Source: CAD feature listing. Evaluate the final solid. Frame: model axes, mm. A direction names the side the tool comes from. Round coordinates to 2 decimals unless told otherwise and drop trailing zeros. Write each loop counter-clockwise with the first axis right and the second up, starting at its lowest first coordinate (ties: lowest second). Pieces come first, ordered by that corner, then holes. Notation, with made-up numbers: M 40.5,-21.5 L 71.5,-21.5 A33 cw 71.5,12.5 Z; hole C -4.5,43.25 d1. An arc over 180 degrees is marked long. Answer in a Markdown table with one row per item.
from build123d import *

# Parameters (mm, degrees)
BOSS_EXTRUDE1_DEPTH = 10
CUT_EXTRUDE1_REACH  = 3.5
SKETCH2_W           = 9
SKETCH2_H           = 5
CUT_EXTRUDE2_REACH  = 4


with BuildPart() as part:
    # Sketch1 → Boss-Extrude1 (new body)
    with BuildSketch(Plane(origin=(0, 0, 0), x_dir=(1, 0, 0), z_dir=(0, 1, 0))):
        Polygon((0, 0), (25.5, 0), (25.5, 11), (24, 11), (24, 2), (10, 2), (10, 14), (0, 14), align=None)
    extrude(amount=BOSS_EXTRUDE1_DEPTH)

    # Sketch2 → Cut-Extrude1 (cut, up to next)
    with BuildSketch(Plane.ZY.offset(-24), mode=Mode.PRIVATE) as cut_extrude1_sk1:
        with Locations((-6.5, 2.5)):
            Rectangle(SKETCH2_W, SKETCH2_H)
    cut_extrude1_tool1 = extrude(cut_extrude1_sk1.sketch, amount=-CUT_EXTRUDE1_REACH, mode=Mode.PRIVATE) & part.part
    add(cut_extrude1_tool1.solids().sort_by_distance((24, 2.5, -6.5))[0], mode=Mode.SUBTRACT)

    # Sketch3 → Cut-Extrude2 (cut, up to next)
    with BuildSketch(Plane(origin=(0, 0, -2), x_dir=(-1, 0, 0), z_dir=(0, 0, -1)), mode=Mode.PRIVATE) as cut_extrude2_sk1:
        with BuildLine():
            Line((-19.5, 5), (-14.5, 5))
            ThreePointArc((-14.5, 5), (-13, 3.5), (-14.5, 2))
            Line((-14.5, 2), (-19.5, 2))
            ThreePointArc((-19.5, 2), (-21, 3.5), (-19.5, 5))
        make_face()
    cut_extrude2_tool1 = extrude(cut_extrude2_sk1.sketch, amount=-CUT_EXTRUDE2_REACH, mode=Mode.PRIVATE) & part.part
    add(cut_extrude2_tool1.solids().sort_by_distance((17, 3.5, -2))[0], mode=Mode.SUBTRACT)


solid = part.part
Q1. Material intervals for probe 1 along X at (y, z) = (7.75, -4.25); probe 2 along Z at (x, y) = (22.75, 5); probe 3 along X at (y, z) = (4, -8.5), sorted ascending.
Solutions:
| item | result |
|---|---|
| probe 1 | x = 0 to 10, 24 to 25.5 |
| probe 2 | z = -2 to 0 |
| probe 3 | x = 0 to 10 |
Q2. Pull-direction query (Y, two-part tool) for faces 5 (the cylindrical face through (21, 3.5, -1)), 6 (the flat face through (7, 0, -7)), 7 (the flat face through (10, 5, -8)); classes: pulls with the +Y half, pulls with the -Y half, needs draft (parallel to the pull), parting line crosses it, or undercut.
Solutions:
| item | result |
|---|---|
| face 5 | undercut |
| face 6 | pulls with the -Y half |
| face 7 | needs draft |
Q3. Access query for faces 1 (the cylindrical face through (13, 3.5, -1)), 2 (the flat face through (25, 7, -11)), 3 (the flat face through (25, 5, -7)), 4 (the flat face through (24, 7, -7)). Directions: +Z, -Z, +X, -X, +Y, -Y. A direction counts if a zero-diameter tool reaches every point of the face in a straight line with its end or side. Return the directions, or none.
Solutions:
| item | result |
|---|---|
| face 1 | +Z, -Z |
| face 2 | -Z, +X, +Y, -Y |
| face 3 | -Z, +X, -Y |
| face 4 | -Z, +Y, -Y |
Q4. Section B-B (y = 3.5). Return loops of the section in (x, z), and give its area (3 significant figures).
Solutions:
| item | result |
|---|---|
| outline | M 0,-14 L 10,-14 L 10,-2 L 13,-2 L 13,0 L 0,0 Z; M 21,-2 L 25.5,-2 L 25.5,0 L 21,0 Z |
| area | 155 mm2 |
Q5. Contact query for flat-ended pins moving along their axis: pin 1 Ø3 at (x, z) = (19, -5) entering from +Y; pin 2 Ø5 at (x, y) = (13.5, 3.5) entering from +Z; pin 3 Ø0.8 at (x, y) = (25, 8) entering from -Z; pin 4 Ø1.6 at (x, z) = (24.5, -6) entering from -Y. Output: stop coordinate, or through.
Solutions:
| item | result |
|---|---|
| pin 1 | passes through |
| pin 2 | stops at z = 0 |
| pin 3 | stops at z = -11 |
| pin 4 | stops at y = 5 |
Q6. Section C-C (x = 17.5). Return loops of the section in (y, z).
Solutions:
| item | result |
|---|---|
| outline | M 0,-2 L 2,-2 L 2,0 L 0,0 Z; M 5,-2 L 10,-2 L 10,0 L 5,0 Z |
Q7. Section A-A (z = -4.75). Return loops of the section in (x, y), and give its area (4 significant figures).
Solutions:
| item | result |
|---|---|
| outline | M 0,0 L 10,0 L 10,10 L 0,10 Z; M 24,5 L 25.5,5 L 25.5,10 L 24,10 Z |
| area | 107.5 mm2 |
Q8. Section D-D (y = 8.25). Return loops of the section in (x, z).
Solutions:
| item | result |
|---|---|
| outline | M 0,-14 L 10,-14 L 10,-2 L 24,-2 L 24,-11 L 25.5,-11 L 25.5,0 L 0,0 Z |
